Design review of the part built by this model. Coordinates are the model's own, in mm. Coordinates: 2 decimals unless noted, no trailing zeros. Order: outer loops, then holes, each group sorted by start corner. A loop starts at its lowest first (then second) coordinate and runs counter-clockwise, first axis right, second up. Notation, with made-up numbers: (-33.5, -26.75) -> (-18.5, -26.75) arc R20 ccw to (-18.5, 3.25) -> close; hole circle Ø11 at (63.5, 48.25). An arc over 180 degrees is marked (long way). Write item = value, one per line.
```python
from build123d import *

# Parameters (mm, degrees)
RESSALTO_EXTRUS_O1_DEPTH = 3
ESBO_O2_W                = 15
ESBO_O2_H                = 30
CORTE_EXTRUS_O1_DEPTH    = 10
ESBO_O3_R                = 2
CORTE_EXTRUS_O2_DEPTH    = 10
ESBO_O4_R                = 2
CORTE_EXTRUS_O3_DEPTH    = 10
ESBO_O5_R                = 2
CORTE_EXTRUS_O4_DEPTH    = 10
ESBO_O6_R                = 2
CORTE_EXTRUS_O5_DEPTH    = 10
ESBO_O7_R                = 6.5
CORTE_EXTRUS_O6_DEPTH    = 10
ESBO_O8_R                = 6.5
CORTE_EXTRUS_O7_DEPTH    = 10


with BuildPart() as part:
    # Esboço1 → Ressalto-extrusão1 (new body)
    with BuildSketch(Plane.XY):
        Polygon((100, 0), (180, 0), (200, 23), (200, 81), (180, 104), (100, 104), (100, 74), (0, 74), (0, 30), (100, 30), align=None)
    extrude(amount=RESSALTO_EXTRUS_O1_DEPTH)

    # Esboço2 → Corte-extrusão1 (cut)
    with BuildSketch(Plane.XY.offset(3)):
        with Locations((116.5, 33.5)):
            Rectangle(ESBO_O2_W, ESBO_O2_H)
    extrude(amount=-CORTE_EXTRUS_O1_DEPTH, mode=Mode.SUBTRACT)

    # Esboço3 → Corte-extrusão2 (cut)
    with BuildSketch(Plane.XY.offset(3)):
        with Locations((109, 4.5)):
            Circle(ESBO_O3_R)
    extrude(amount=-CORTE_EXTRUS_O2_DEPTH, mode=Mode.SUBTRACT)

    # Esboço4 → Corte-extrusão3 (cut)
    with BuildSketch(Plane.XY.offset(3)):
        with Locations((175.5, 7.5)):
            Circle(ESBO_O4_R)
    extrude(amount=-CORTE_EXTRUS_O3_DEPTH, mode=Mode.SUBTRACT)

    # Esboço5 → Corte-extrusão4 (cut)
    with BuildSketch(Plane.XY.offset(3)):
        with Locations((108, 97.7)):
            Circle(ESBO_O5_R)
    extrude(amount=-CORTE_EXTRUS_O4_DEPTH, mode=Mode.SUBTRACT)

    # Esboço6 → Corte-extrusão5 (cut)
    with BuildSketch(Plane.XY.offset(3)):
        with Locations((174.5, 99)):
            Circle(ESBO_O6_R)
    extrude(amount=-CORTE_EXTRUS_O5_DEPTH, mode=Mode.SUBTRACT)

    # Esboço7 → Corte-extrusão6 (cut)
    with BuildSketch(Plane.XY.offset(3)):
        with Locations((181.63, 86.5)):
            Circle(ESBO_O7_R)
        with Locations((181.63, 17.5)):
            Circle(ESBO_O7_R)
    extrude(amount=-CORTE_EXTRUS_O6_DEPTH, mode=Mode.SUBTRACT)

    # Esboço8 → Corte-extrusão7 (cut)
    with BuildSketch(Plane.XY.offset(3)):
        with Locations((189.996600265, 52)):
            Circle(ESBO_O8_R)
    extrude(amount=-CORTE_EXTRUS_O7_DEPTH, mode=Mode.SUBTRACT)


solid = part.part
```
(1) We need section B-B (z = 0.75). Give the number of separate pieces and of enclosed holes in the cut face, and give its area (3 significant figures).
Report:
separate_pieces = 1
enclosed_holes = 8
area = 13,400 mm²
(2) We need section D-D (y = 86.5). Write out the cut boundary in (x, z).
Report:
outline = (100, 0) -> (175.13, 0) -> (175.13, 3) -> (100, 3) -> close; (188.13, 0) -> (195.22, 0) -> (195.22, 3) -> (188.13, 3) -> close
(3) The part is to be moulded in two halves that separate along X. For faces 1 (the cylindrical face through (107.002, 4.588, 1.521)), 2 (the flat face through (121, 53, 3)), 3 (the flat face through (189.86, 11.34, 1.48)), say which applies: released by +X, released by -X, zero draft, split by the parting line, or undercut.
Report:
face_1 = undercut
face_2 = zero draft
face_3 = released by +X
(4) Insertion check: pin 1 (1.5 mm diameter, centred on x = 28, z = 2, fed in from +Y); pin 2 (1.5 mm diameter, centred on x = 69.5, z = 1, fed in from -Y); pin 3 (21 mm diameter, centred on x = 181.63, y = 86.5, fed in from +Z); pin 4 (1.5 mm diameter, centred on y = 85.5, z = 1, fed in from -X). Each pin has a flat end and moves straight along its axis. Give the tip position at first contact, or say it passes through.
Report:
pin_1 = 74
pin_2 = 30
pin_3 = 3
pin_4 = 100
(5) For L1, parallel to Y at x = 181.63, z = 0.9; L2, parallel to X at y = 29.5, z = 0.3; L3, parallel to X at y = 47, z = 0.3, list the stretches that pass through material, from the lowest coordinate up.
Report:
L1 = 1.87 to 11, 24 to 80, 93 to 102.13
L2 = 100 to 109, 124 to 200
L3 = 0 to 109, 124 to 185.84, 194.15 to 200
(6) We need section C-C (x = 42.5). Write out the cut boundary in (y, z).
Report:
outline = (30, 0) -> (74, 0) -> (74, 3) -> (30, 3) -> close
(7) We need section A-A (y = 52). Write out the cut boundary in (x, z).
Report:
outline = (0, 0) -> (183.5, 0) -> (183.5, 3) -> (0, 3) -> close; (196.5, 0) -> (200, 0) -> (200, 3) -> (196.5, 3) -> close
